from build123d import *

# Parameters (mm, degrees)
SKETCH2_R          = 33.3375
SKETCH3_R          = 23.8125
CUT_EXTRUDE1_DEPTH = 256.54
SKETCH4_R          = 23.8125
CUT_EXTRUDE2_DEPTH = 261.62


with BuildPart() as part:
    # Sweep1: sweep along a path in Sketch1
    with BuildLine(Plane.XY) as sweep1_path:
        Line((0, 0), (0, 266.7))
        ThreePointArc((0, 266.7), (59.515902063, 410.384097937), (203.2, 469.9))
        Line((203.2, 469.9), (406.4, 469.9))
        ThreePointArc((406.4, 469.9), (550.084097937, 410.384097937), (609.6, 266.7))
        Line((609.6, 266.7), (609.6, 0))
    # Sketch2 → Sweep1 (sweep)
    with BuildSketch(Plane(origin=(0, 0, 0), x_dir=(1, 0, 0), z_dir=(0, 1, 0))):
        Circle(SKETCH2_R)
    sweep(path=sweep1_path.line)

    # Sketch3 → Cut-Extrude1 (cut)
    with BuildSketch(Plane.XZ):
        with Locations(Location((0, 0, 0), (0, 0, 270))):
            Circle(SKETCH3_R)
    extrude(amount=-CUT_EXTRUDE1_DEPTH, mode=Mode.SUBTRACT)

    # Sketch4 → Cut-Extrude2 (cut)
    with BuildSketch(Plane.XZ):
        with Locations((609.6, 0)):
            Circle(SKETCH4_R)
    extrude(amount=-CUT_EXTRUDE2_DEPTH, mode=Mode.SUBTRACT)


solid = part.part
Can you work these out from the model? Positions are in its coordinate system, mm. A direction names the side the tool comes from. Coordinates: 2 decimals unless noted, no trailing zeros. Write each loop counter-clockwise with the first axis right and the second up, starting at its lowest first coordinate (ties: lowest second). Pieces come first, ordered by that corner, then holes. Notation, with made-up numbers: M -17,4 L -2,4 A24 cw -2,20 Z; hole C 86,17 d4. An arc over 180 degrees is marked long. Use one line per item in the form item = value.
Q1. For P1, Ø14.5, axis at x = 617, z = -2.5, coming from the -Y side; P2, Ø4, axis at x = 391.5, z = 1.5, coming from the -Y side; P3, Ø8, axis at x = 345, z = 20.5, coming from the +Y side, each with a flat end and sliding along its axis, tell me the tip position at first contact or that it passes through.
Model answer:
P1 = 261.62
P2 = 436.56
P3 = 498.87
Q2. I need wall thicknesses on line 1 along X through (y, z) = (34, 2); line 2 along Z through (x, y) = (609.6, 73); line 3 along X through (y, z) = (175, 2.5). Which ranges of each line are inside material? Lowest first, please. Write a range as from..to.
Model answer:
line_1 = -33.28..-23.73, 23.73..33.28, 576.32..585.87, 633.33..642.88
line_2 = -33.34..-23.81, 23.81..33.34
line_3 = -33.24..-23.68, 23.68..33.24, 576.36..585.92, 633.28..642.84
Q3. If we section it at C-C (x = 389.5): Write out the boundary of the cut face in (y, z) (1 decimal).
Model answer:
outline = C 469.9,0 d66.7
Q4. If we section it at B-B (y = 114): Write out the boundary of the cut face in (x, z) (1 decimal), then the cut area to 3 significant figures.
Model answer:
outline = C 0,0 d66.7; C 609.6,0 d66.7; hole C 0,0 d47.6; hole C 609.6,0 d47.6
area = 3,420 mm^2
Q5. For faces 4 (the cylindrical face through (306.222, 503.205, -1.466)), 5 (the flat face through (617, 0, 23)), 6 (the cylindrical face through (31.8, 135.22, -10.01)), which set-ups out of +Z, -Z, +X, -X, +Y, -Y let a thin tool reach every point of the face, with its end or its side?
Model answer:
face_4 = none
face_5 = +Z, -Z, +X, -X, -Y
face_6 = -Y
Q6. We'd pull the mould along Z, two halves only. Please class faces 1 (the cylindrical face through (578.805, 131.483, 12.768)), 2 (the flat face through (609, 261.62, 0)), 3 (the flat face through (23, 0, -8)): +Z half, -Z half, draft (parallel to the pull), parting line (faces both ways), or undercut.
Model answer:
face_1 = parting line
face_2 = undercut
face_3 = draft
Q7. If we section it at A-A (z = 0): Write out the boundary of the cut face in (x, y) (1 decimal), then the cut area to 3 significant figures.
Model answer:
outline = M -33.3,0 L -23.8,0 L -23.8,256.5 L 23.8,256.5 L 23.8,0 L 33.3,0 L 33.3,266.7 A169.9 cw 203.2,436.6 L 406.4,436.6 A169.9 cw 576.3,266.7 L 576.3,0 L 585.8,0 L 585.8,261.6 L 633.4,261.6 L 633.4,0 L 642.9,0 L 642.9,266.7 A236.5 ccw 406.4,503.2 L 203.2,503.2 A236.5 ccw -33.3,266.7 Z
area = 67,000 mm^2
